Verification items for the finished model (mm, model axes). Face numbers are marked on the shaded views. A direction names the side the tool comes from. Round coordinates to 2 decimals unless told otherwise and drop trailing zeros. Loops run counter-clockwise (first coordinate to the right, second up) from the corner with the lowest first, then second, coordinate; pieces in that order, holes last. Notation, with made-up numbers: M 50,2 L 93,2 A19 ccw 93,10 Z; hole C 62.25,28 d6. An arc over 180 degrees is marked long. Write item = value, one per line. Start each with the question number.
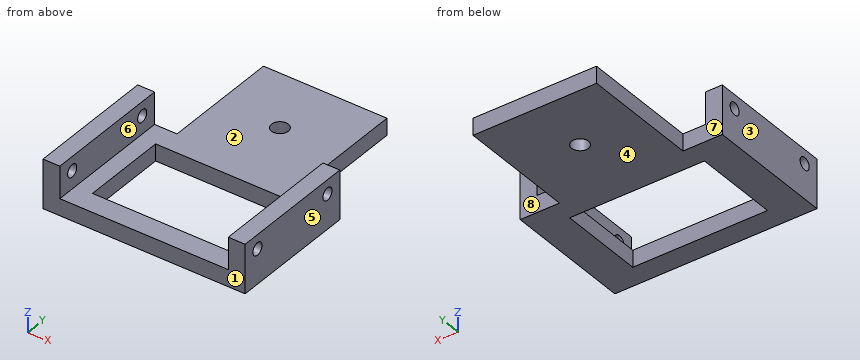
from build123d import *

# Parameters (mm, degrees)
SKETCH1_W           = 24
SKETCH1_H           = 15.333333334
SKETCH1_R           = 1.5
BOSS_EXTRUDE1_DEPTH = 3
SKETCH1_4_W         = 3
SKETCH1_4_H         = 23
BOSS_EXTRUDE2_DEPTH = 8.7
CUT_EXTRUDE1_REACH  = 51.274
SKETCH2_R           = 1.1


with BuildPart() as part:
    # Sketch1 → Boss-Extrude1 (new body)
    with BuildSketch(Plane.XY):
        Polygon((-11, 32.5), (-11, 11.5), (-15, 11.5), (-15, -11.5), (15, -11.5), (15, 11.5), (11, 11.5), (11, 32.5), align=None)
        Rectangle(SKETCH1_W, SKETCH1_H, mode=Mode.SUBTRACT)
        with Locations((0, 21.5)):
            Circle(SKETCH1_R, mode=Mode.SUBTRACT)
    extrude(amount=BOSS_EXTRUDE1_DEPTH)

    # Sketch1<4> → Boss-Extrude2 (add)
    with BuildSketch(Plane.XY):
        with Locations((16.5, 0)):
            Rectangle(SKETCH1_4_W, SKETCH1_4_H)
        with Locations((-16.5, 0)):
            Rectangle(SKETCH1_4_W, SKETCH1_4_H)
    extrude(amount=BOSS_EXTRUDE2_DEPTH)

    # Cut-Extrude1: up to this face of the body (flat: up to its plane)
    cut_extrude1_end = Plane(part.part.faces().sort_by_distance((-18, 0, 4.35))[0])
    # Sketch2 → Cut-Extrude1 (cut, up to the picked face)
    with BuildSketch(Plane(origin=(18, 0, 0), x_dir=(0, 0, -1), z_dir=(1, 0, 0)), mode=Mode.PRIVATE) as cut_extrude1_sk1:
        with Locations(Location((-6.2, 8.5, 0), (0, 0, 90))):
            Circle(SKETCH2_R)
    cut_extrude1_tool1 = split(extrude(cut_extrude1_sk1.sketch, amount=-CUT_EXTRUDE1_REACH, mode=Mode.PRIVATE), bisect_by=cut_extrude1_end, keep=Keep.BOTH, mode=Mode.PRIVATE)
    # Sketch2 → Cut-Extrude1 (cut, up to the picked face)
    with BuildSketch(Plane(origin=(18, 0, 0), x_dir=(0, 0, -1), z_dir=(1, 0, 0)), mode=Mode.PRIVATE) as cut_extrude1_sk2:
        with Locations(Location((-6.2, -8.5, 0), (0, 0, 90))):
            Circle(SKETCH2_R)
    cut_extrude1_tool2 = split(extrude(cut_extrude1_sk2.sketch, amount=-CUT_EXTRUDE1_REACH, mode=Mode.PRIVATE), bisect_by=cut_extrude1_end, keep=Keep.BOTH, mode=Mode.PRIVATE)
    add(cut_extrude1_tool1.solids().sort_by(Axis((18, 8.5, 6.2), (-1, 0, 0)))[0], mode=Mode.SUBTRACT)
    add(cut_extrude1_tool2.solids().sort_by(Axis((18, -8.5, 6.2), (-1, 0, 0)))[0], mode=Mode.SUBTRACT)


solid = part.part
1. Section check C-C, the plane z = 6.2. Enter the section's corners in (x, y), and give its area (3 significant figures).
2. Section check B-B, the plane x = 0. Enter the section's corners in (y, z).
3. Gauge pin test, flat ends, axial feed: P1, Ø1, axis at x = 5, y = 27.5, coming from the +Z side; P2, Ø3.5, axis at y = 19.5, z = 2, coming from the -X side; P3, Ø3.5, axis at y = 21, z = 2, coming from the +X side. Record the tip position at first contact, or that the pin passes through.
4. Mould release check, pull along X, two halves, no side actions. Record for the marked faces 1, 2 and 3: pulls with the +X half, pulls with the -X half, needs draft (parallel to the pull), parting line crosses it, or undercut.
5. Thickness scan on line 1 (Y direction, x = 0, z = 1.2); line 2 (Y direction, x = -6.5, z = 1.5); line 3 (X direction, y = 2.5, z = 4.5). Record the ranges inside material, lowest first.
6. Tool access check on the marked faces 4, 5, 6, 7 and 8. Record the directions out of +Z, -Z, +X, -X, +Y, -Y that give a thin tool (end or side, any length) a straight path to the whole face; none if there is none.
7. Section check A-A, the plane y = 21.5. Enter the section's corners in (x, z), and give its area (3 significant figures).
8. Section check D-D, the plane y = 8.5. Enter the section's corners in (x, z), and give its area (3 significant figures).
Computed values:
q1.outline = M -18,-11.5 L -15,-11.5 L -15,-9.6 L -18,-9.6 Z; M -18,-7.4 L -15,-7.4 L -15,7.4 L -18,7.4 Z; M -18,9.6 L -15,9.6 L -15,11.5 L -18,11.5 Z; M 15,-11.5 L 18,-11.5 L 18,-9.6 L 15,-9.6 Z; M 15,-7.4 L 18,-7.4 L 18,7.4 L 15,7.4 Z; M 15,9.6 L 18,9.6 L 18,11.5 L 15,11.5 Z
q1.area = 112 mm2
q2.outline = M -11.5,0 L -7.67,0 L -7.67,3 L -11.5,3 Z; M 7.67,0 L 20,0 L 20,3 L 7.67,3 Z; M 23,0 L 32.5,0 L 32.5,3 L 23,3 Z
q3.P1 = 3
q3.P2 = -11
q3.P3 = 11
q4.face_1 = needs draft
q4.face_2 = undercut
q4.face_3 = pulls with the -X half
q5.line_1 = -11.5 to -7.67, 7.67 to 20, 23 to 32.5
q5.line_2 = -11.5 to -7.67, 7.67 to 32.5
q5.line_3 = -18 to -15, 15 to 18
q6.face_4 = -Z, +X, -X, +Y, -Y
q6.face_5 = +Z, -Z, +X, +Y, -Y
q6.face_6 = +Z, +Y, -Y
q6.face_7 = +Z, -Z, -X, +Y
q6.face_8 = +Z, -Z, +X, +Y
q7.outline = M -11,0 L -1.5,0 L -1.5,3 L -11,3 Z; M 1.5,0 L 11,0 L 11,3 L 1.5,3 Z
q7.area = 57.0 mm2
q8.outline = M -18,0 L 18,0 L 18,5.1 L 15,5.1 L 15,3 L -15,3 L -15,5.1 L -18,5.1 Z; M -18,7.3 L -15,7.3 L -15,8.7 L -18,8.7 Z; M 15,7.3 L 18,7.3 L 18,8.7 L 15,8.7 Z
q8.area = 129 mm2
